from build123d import *

# Parameters (mm, degrees)
SKETCH_1_W          = 197
SKETCH_1_H          = 229
EXTRUDE_1_DEPTH     = 2.7
SKETCH_2_R          = 1.1
CUT_EXTRUDE_1_DEPTH = 2.85
SKETCH_6_W          = 20
SKETCH_6_H          = 80
SKETCH_6_H_2        = 150
CUT_EXTRUDE_4_DEPTH = 10
FILLET_1_R          = 5
SKETCH_7_R          = 1.25
CUT_EXTRUDE_5_DEPTH = 10


with BuildPart() as part:
    # 草图1 → 凸台-拉伸1 (new body)
    with BuildSketch(Plane.XY):
        with Locations((98.5, 114.5)):
            Rectangle(SKETCH_1_W, SKETCH_1_H)
    extrude(amount=EXTRUDE_1_DEPTH)

    # 草图2 → 切除-拉伸1 (cut)
    with BuildSketch(Plane.XY.offset(2.7)):
        with Locations((4, 4)):
            Circle(SKETCH_2_R)
        with Locations((193, 4)):
            Circle(SKETCH_2_R)
    extrude(amount=-CUT_EXTRUDE_1_DEPTH, mode=Mode.SUBTRACT)

    # 草图6 → 切除-拉伸4 (cut)
    with BuildSketch(Plane(origin=(0, 0, 0), x_dir=(-1, 0, 0), z_dir=(0, 0, -1))):
        with Locations((-168.5, 114.5)):
            Rectangle(SKETCH_6_W, SKETCH_6_H)
        with Locations((-28.5, 114.5)):
            Rectangle(SKETCH_6_W, SKETCH_6_H)
        with Locations((-98.5, 114.5)):
            Rectangle(SKETCH_6_W, SKETCH_6_H_2)
    extrude(amount=-CUT_EXTRUDE_4_DEPTH, mode=Mode.SUBTRACT)

    # 圆角1
    fillet_1_edges = [part.edges().sort_by_distance(p)[0] for p in [
        (178.5, 74.5, 1.35),
        (178.5, 154.5, 1.35),
        (158.5, 154.5, 1.35),
        (158.5, 74.5, 1.35),
        (38.5, 74.5, 1.35),
        (38.5, 154.5, 1.35),
        (18.5, 154.5, 1.35),
        (18.5, 74.5, 1.35),
        (108.5, 39.5, 1.35),
        (108.5, 189.5, 1.35),
        (88.5, 189.5, 1.35),
        (88.5, 39.5, 1.35),
    ]]
    fillet(fillet_1_edges, radius=FILLET_1_R)

    # 草图7 → 切除-拉伸5 (cut)
    with BuildSketch(Plane.XY.offset(2.7)):
        with Locations((76, 184)):
            Circle(SKETCH_7_R)
        with Locations((121, 184)):
            Circle(SKETCH_7_R)
        with Locations((76, 139)):
            Circle(SKETCH_7_R)
        with Locations((121, 139)):
            Circle(SKETCH_7_R)
        with Locations(Location((121, 90, 0), (0, 0, 180))):
            Circle(SKETCH_7_R)
        with Locations(Location((76, 90, 0), (0, 0, 180))):
            Circle(SKETCH_7_R)
        with Locations(Location((121, 45, 0), (0, 0, 180))):
            Circle(SKETCH_7_R)
        with Locations(Location((76, 45, 0), (0, 0, 180))):
            Circle(SKETCH_7_R)
    extrude(amount=-CUT_EXTRUDE_5_DEPTH, mode=Mode.SUBTRACT)


solid = part.part
Could you check a few things on this model? Use its own coordinates, in mm. A direction names the side the tool comes from. Give positions to 0.01 mm unless a question says otherwise; leave off trailing zeros. Loops run counter-clockwise (first coordinate to the right, second up) from the corner with the lowest first, then second, coordinate; pieces in that order, holes last. Notation, with made-up numbers: M -9.5,57 L -2.5,57 A33 cw -2.5,85 Z; hole C 52,20 d5. An arc over 180 degrees is marked long. Answer as a JSON object with one key per item and string values.
Q1. For P1, Ø1, axis at x = 76, z = 2, coming from the -Y side, with a flat end and sliding along its axis, tell me the tip position at first contact or that it passes through.
Values found:
{"P1": "stops at y = 0"}
Q2. Suppose I cut it at B-B, the plane y = 119. List the corners of the cut face in (x, z) for me, plus the area to 3 significant figures.
Values found:
{"outline": "M 0,0 L 18.5,0 L 18.5,2.7 L 0,2.7 Z; M 38.5,0 L 88.5,0 L 88.5,2.7 L 38.5,2.7 Z; M 108.5,0 L 158.5,0 L 158.5,2.7 L 108.5,2.7 Z; M 178.5,0 L 197,0 L 197,2.7 L 178.5,2.7 Z", "area": "370 mm²"}
Q3. For faces 1 (the flat face through (119, 116, 2.7)), 2 (the cylindrical face through (160, 153.07, 1.37)), which set-ups out of +Z, -Z, +X, -X, +Y, -Y let a thin tool reach every point of the face, with its end or its side?
Values found:
{"face 1": "+Z, +X, -X, +Y, -Y", "face 2": "+Z, -Z"}
Q4. If we mould it in two halves opening along X, with no side actions, what happens to faces 3 (the cylindrical face through (107.07, 41, 1.37)), 4 (the flat face through (119, 116, 0))? For each: pulls with the +X half, pulls with the -X half, needs draft (parallel to the pull), parting line crosses it, or undercut.
Values found:
{"face 3": "undercut", "face 4": "needs draft"}
Q5. Suppose I cut it at A-A, the plane x = 29.5. List the corners of the cut face in (y, z) for me.
Values found:
{"outline": "M 0,0 L 74.5,0 L 74.5,2.7 L 0,2.7 Z; M 154.5,0 L 229,0 L 229,2.7 L 154.5,2.7 Z"}
Q6. If I drill on probe 1 along Y at (x, z) = (76, 1.2); probe 2 along X at (y, z) = (139, 1.1); probe 3 along X at (y, z) = (87.5, 0.6), over which ranges is the centre line in solid material (lowest first)? Write a range as [from, to].
Values found:
{"probe 1": "y = [0, 43.75], [46.25, 88.75], [91.25, 137.75], [140.25, 182.75], [185.25, 229]", "probe 2": "x = [0, 18.5], [38.5, 74.75], [77.25, 88.5], [108.5, 119.75], [122.25, 158.5], [178.5, 197]", "probe 3": "x = [0, 18.5], [38.5, 88.5], [108.5, 158.5], [178.5, 197]"}
